Could you check a few things on this model? Use its own coordinates, in mm. A direction names the side the tool comes from. Round coordinates to 2 decimals unless told otherwise and drop trailing zeros. Write each loop counter-clockwise with the first axis right and the second up, starting at its lowest first coordinate (ties: lowest second). Pieces come first, ordered by that corner, then holes. Notation, with made-up numbers: (-15, 49.5) -> (0, 49.5) arc R5 ccw to (0, 56.5) -> close; hole circle Ø4 at (54, 45.25). An arc over 180 degrees is marked (long way). Answer as CSV lines item,"result". Start each with the question number.
Q1. Imagine slicing it at A-A on x = -23.25. Please give me the cut outline in (y, z).
Q2. For faces 1 (the cylindrical face through (39.43, 24.82, 20.07)), 2 (the cylindrical face through (-28.319, -28.778, 29.944)), 3 (the flat face through (-68.2, 0, -46)), which set-ups out of +Z, -Z, +X, -X, +Y, -Y let a thin tool reach every point of the face, with its end or its side?
Q3. Will these pins go through, and if not, where does the flat tip stop? pin 1 Ø19.5 at (x, y) = (23.25, 23.25) entering from -Z; pin 2 Ø9 at (x, z) = (42.5, -4.2) entering from +Y; pin 3 Ø7 at (x, y) = (-23.25, -23.25) entering from +Z; pin 4 Ø7.5 at (y, z) = (23.25, -63) entering from -X.
Q4. If we mould it in two halves opening along Y, with no side actions, what happens to faces 4 (the cylindrical face through (59.243, 22.53, -24.456)), 5 (the flat face through (68.2, 0, 51)), 6 (the cylindrical face through (-59, 26.32, 20.07)), 7 (the conical face through (-42.183, 13.562, -4.698))? For each: pulls with the +Y half, pulls with the -Y half, needs draft (parallel to the pull), parting line crosses it, or undercut.
Q5. Imagine slicing it at B-B on x = -57. Give the number of separate pieces and of enclosed holes in the cut face, and give its area (3 significant figures).
Q6. If I drill on line 1 (Y direction, x = 23.25, z = 19); line 2 (Z direction, x = 58, y = -23.25); line 3 (Z direction, x = -42, y = 20), over which ranges is the centre line in solid material (lowest first)? Write a range as [from, to].
Q7. Imagine slicing it at C-C on x = -7.5. Please give me the cut outline in (y, z).
from build123d import *

# Parameters (mm, degrees)
BOSS_EXTRUDE1_DEPTH      = 35
BOSS_EXTRUDE1_DEPTH_BACK = 35
SKETCH2_W                = 36
SKETCH2_H                = 20
HOLE1_D                  = 6.647
HOLE1_DEPTH              = 19.414509714
HOLE1_CSINK_D            = 8
HOLE1_CSINK_ANGLE        = 90
HOLE1_TIP                = 1.91882362
HOLE2_D                  = 6.647
HOLE2_DEPTH              = 19.414509714
HOLE2_CSINK_D            = 8
HOLE2_CSINK_ANGLE        = 90
HOLE2_TIP                = 1.91882362
HOLE3_D                  = 6.647
HOLE3_DEPTH              = 19.414509714
HOLE3_CSINK_D            = 8
HOLE3_CSINK_ANGLE        = 90
HOLE3_TIP                = 1.91882362
SKETCH26_R               = 10
CUT_EXTRUDE1_DEPTH       = 150
SKETCH27_R               = 10
CUT_EXTRUDE2_DEPTH       = 150
SKETCH28_W               = 177
SKETCH28_H               = 190
CUT_EXTRUDE3_DEPTH       = 70
CUT_EXTRUDE3_DEPTH_BACK  = 70
SKETCH29_R               = 4
CUT_EXTRUDE4_DEPTH       = 17.5
M8_TAPPED_HOLE1_D        = 6.8
M8_TAPPED_HOLE1_DEPTH    = 19.75
M8_TAPPED_HOLE1_TIP      = 2.042926105


with BuildPart() as part:
    # Sketch1 → Boss-Extrude1 (new body, two sides)
    with BuildSketch(Plane(origin=(0, 0, 0), x_dir=(1, 0, 0), z_dir=(0, 1, 0))) as boss_extrude1_sk:
        with BuildLine():
            Line((-68.5, -71), (-35.25, -71))
            Line((-35.25, -71), (-35.25, -34))
            Line((-35.25, -34), (35.25, -34))
            Line((35.25, -34), (35.25, -71))
            Line((35.25, -71), (68.5, -71))
            Line((68.5, -71), (68.5, 79))
            Line((68.5, 79), (35.25, 79))
            Line((35.25, 79), (35.25, 0))
            ThreePointArc((35.25, 0), (34, -1.25), (32.75, 0))
            Line((32.75, 0), (-32.75, 0))
            ThreePointArc((-32.75, 0), (-34, -1.25), (-35.25, 0))
            Line((-35.25, 0), (-35.25, 79))
            Line((-35.25, 79), (-68.5, 79))
            Line((-68.5, 79), (-68.5, -71))
        make_face()
    extrude(amount=BOSS_EXTRUDE1_DEPTH)
    extrude(boss_extrude1_sk.sketch, amount=-BOSS_EXTRUDE1_DEPTH_BACK)

    # Sketch2 → Cut-Revolve1 (revolve, cut)
    with BuildSketch(Plane(origin=(0, 0, 0), x_dir=(0, 0, -1), z_dir=(1, 0, 0))):
        with Locations((-17, 10)):
            Rectangle(SKETCH2_W, SKETCH2_H)
    revolve(axis=Axis((0, 0, -1), (0, 0, 1)), mode=Mode.SUBTRACT)

    # Sketch3 → Cut-Revolve2 (revolve, cut)
    with BuildSketch(Plane(origin=(-23.25, 0, 0), x_dir=(0, 0, -1), z_dir=(1, 0, 0))):
        Polygon((-34, 23.25), (-34, 30.75), (-26, 30.75), (-26, 27.75), (0, 27.75), (0, 23.25), align=None)
    revolve(axis=Axis((-23.25, 23.25, 0), (0, 0, 1)), mode=Mode.SUBTRACT)

    # Sketch4 → Cut-Revolve3 (revolve, cut)
    with BuildSketch(Plane(origin=(-23.25, 0, 0), x_dir=(0, 0, -1), z_dir=(1, 0, 0))):
        Polygon((-34, -23.25), (-34, -15.75), (-26, -15.75), (-26, -18.75), (0, -18.75), (0, -23.25), align=None)
    revolve(axis=Axis((-23.25, -23.25, 0), (0, 0, 1)), mode=Mode.SUBTRACT)

    # Sketch5 → Cut-Revolve4 (revolve, cut)
    with BuildSketch(Plane(origin=(23.25, 0, 0), x_dir=(0, 0, -1), z_dir=(1, 0, 0))):
        Polygon((-34, 23.25), (-34, 30.75), (-26, 30.75), (-26, 27.75), (0, 27.75), (0, 23.25), align=None)
    revolve(axis=Axis((23.25, 23.25, 0), (0, 0, 1)), mode=Mode.SUBTRACT)

    # Sketch6 → Cut-Revolve5 (revolve, cut)
    with BuildSketch(Plane(origin=(23.25, 0, 0), x_dir=(0, 0, -1), z_dir=(1, 0, 0))):
        Polygon((-34, -23.25), (-34, -15.75), (-26, -15.75), (-26, -18.75), (0, -18.75), (0, -23.25), align=None)
    revolve(axis=Axis((23.25, -23.25, 0), (0, 0, 1)), mode=Mode.SUBTRACT)

    # Hole1
    with Locations(Plane(origin=(0, 35, 0), x_dir=(1, 0, 0), z_dir=(0, 1, 0))):
        with Locations((42.5, -18.8)):
            CounterSinkHole(HOLE1_D / 2, HOLE1_CSINK_D / 2, depth=HOLE1_DEPTH, counter_sink_angle=HOLE1_CSINK_ANGLE)
            with Locations((0, 0, -(HOLE1_DEPTH + HOLE1_TIP / 2))):  # 120° drill point
                Cone(0, HOLE1_D / 2, HOLE1_TIP, mode=Mode.SUBTRACT)

    # Hole2
    with Locations(Plane(origin=(0, 35, 0), x_dir=(1, 0, 0), z_dir=(0, 1, 0))):
        with Locations((-42.5, -18.8)):
            CounterSinkHole(HOLE2_D / 2, HOLE2_CSINK_D / 2, depth=HOLE2_DEPTH, counter_sink_angle=HOLE2_CSINK_ANGLE)
            with Locations((0, 0, -(HOLE2_DEPTH + HOLE2_TIP / 2))):  # 120° drill point
                Cone(0, HOLE2_D / 2, HOLE2_TIP, mode=Mode.SUBTRACT)

    # Sketch11 → Cut-Revolve6 (revolve, cut)
    with BuildSketch(Plane.XY.offset(18.8)):
        Polygon((48.5, 23.25), (50.41882362, 26.5735), (67.8235, 26.5735), (68.5, 27.25), (68.5, 23.25), align=None)
    revolve(axis=Axis((68.5, 23.25, 18.8), (-1, 0, 0)), mode=Mode.SUBTRACT)

    # Sketch12 → Cut-Revolve7 (revolve, cut)
    with BuildSketch(Plane.XY.offset(18.8)):
        Polygon((48.5, -23.25), (50.41882362, -19.9265), (67.8235, -19.9265), (68.5, -19.25), (68.5, -23.25), align=None)
    revolve(axis=Axis((68.5, -23.25, 18.8), (-1, 0, 0)), mode=Mode.SUBTRACT)

    # Sketch13 → Cut-Revolve8 (revolve, cut)
    with BuildSketch(Plane.XY.offset(18.8)):
        Polygon((-68.5, 23.25), (-68.5, 27.25), (-67.8235, 26.5735), (-50.41882362, 26.5735), (-48.5, 23.25), align=None)
    revolve(axis=Axis((-48.5, 23.25, 18.8), (-1, 0, 0)), mode=Mode.SUBTRACT)

    # Sketch14 → Cut-Revolve9 (revolve, cut)
    with BuildSketch(Plane.XY.offset(18.8)):
        Polygon((-68.5, -23.25), (-68.5, -19.25), (-67.8235, -19.9265), (-50.41882362, -19.9265), (-48.5, -23.25), align=None)
    revolve(axis=Axis((-48.5, -23.25, 18.8), (-1, 0, 0)), mode=Mode.SUBTRACT)

    # Hole3
    with Locations(Plane(origin=(0, 35, 0), x_dir=(1, 0, 0), z_dir=(0, 1, 0))):
        with Locations((42.5, 27.7)):
            CounterSinkHole(HOLE3_D / 2, HOLE3_CSINK_D / 2, depth=HOLE3_DEPTH, counter_sink_angle=HOLE3_CSINK_ANGLE)
            with Locations((0, 0, -(HOLE3_DEPTH + HOLE3_TIP / 2))):  # 120° drill point
                Cone(0, HOLE3_D / 2, HOLE3_TIP, mode=Mode.SUBTRACT)

    # Sketch17 → Cut-Revolve10 (revolve, cut)
    with BuildSketch(Plane.XY.offset(-27.7)):
        Polygon((-42.5, 35), (-38.5, 35), (-39.1765, 34.3235), (-39.1765, 15.585490286), (-42.5, 13.666666667), align=None)
    revolve(axis=Axis((-42.5, 13.666666667, -27.7), (0, 1, 0)), mode=Mode.SUBTRACT)

    # Sketch18 → Cut-Revolve11 (revolve, cut)
    with BuildSketch(Plane.XY.offset(-27.7)):
        Polygon((48.5, 23.25), (50.41882362, 26.5735), (67.8235, 26.5735), (68.5, 27.25), (68.5, 23.25), align=None)
    revolve(axis=Axis((68.5, 23.25, -27.7), (-1, 0, 0)), mode=Mode.SUBTRACT)

    # Sketch19 → Cut-Revolve12 (revolve, cut)
    with BuildSketch(Plane.XY.offset(-27.7)):
        Polygon((48.5, -23.25), (50.41882362, -19.9265), (67.8235, -19.9265), (68.5, -19.25), (68.5, -23.25), align=None)
    revolve(axis=Axis((68.5, -23.25, -27.7), (-1, 0, 0)), mode=Mode.SUBTRACT)

    # Sketch20 → Cut-Revolve13 (revolve, cut)
    with BuildSketch(Plane.XY.offset(-27.7)):
        Polygon((-68.5, 23.25), (-68.5, 27.25), (-67.8235, 26.5735), (-50.41882362, 26.5735), (-48.5, 23.25), align=None)
    revolve(axis=Axis((-48.5, 23.25, -27.7), (-1, 0, 0)), mode=Mode.SUBTRACT)

    # Sketch21 → Cut-Revolve14 (revolve, cut)
    with BuildSketch(Plane.XY.offset(-27.7)):
        Polygon((-68.5, -23.25), (-68.5, -19.25), (-67.8235, -19.9265), (-50.41882362, -19.9265), (-48.5, -23.25), align=None)
    revolve(axis=Axis((-48.5, -23.25, -27.7), (-1, 0, 0)), mode=Mode.SUBTRACT)

    # Sketch22 → Cut-Revolve15 (revolve, cut)
    with BuildSketch(Plane.XY.offset(-63)):
        Polygon((-68.5, 23.25), (-68.5, 27.25), (-67.8235, 26.5735), (-50.41882362, 26.5735), (-48.5, 23.25), align=None)
    revolve(axis=Axis((-48.5, 23.25, -63), (-1, 0, 0)), mode=Mode.SUBTRACT)

    # Sketch23 → Cut-Revolve16 (revolve, cut)
    with BuildSketch(Plane.XY.offset(-63)):
        Polygon((-68.5, -23.25), (-68.5, -19.25), (-67.8235, -19.9265), (-50.41882362, -19.9265), (-48.5, -23.25), align=None)
    revolve(axis=Axis((-48.5, -23.25, -63), (-1, 0, 0)), mode=Mode.SUBTRACT)

    # Sketch24 → Cut-Revolve17 (revolve, cut)
    with BuildSketch(Plane.XY.offset(37)):
        Polygon((-68.5, 23.25), (-68.5, 27.25), (-67.8235, 26.5735), (-50.41882362, 26.5735), (-48.5, 23.25), align=None)
    revolve(axis=Axis((-48.5, 23.25, 37), (-1, 0, 0)), mode=Mode.SUBTRACT)

    # Sketch25 → Cut-Revolve18 (revolve, cut)
    with BuildSketch(Plane.XY.offset(37)):
        Polygon((-68.5, -23.25), (-68.5, -19.25), (-67.8235, -19.9265), (-50.41882362, -19.9265), (-48.5, -23.25), align=None)
    revolve(axis=Axis((-48.5, -23.25, 37), (-1, 0, 0)), mode=Mode.SUBTRACT)

    # Sketch26 → Cut-Extrude1 (cut)
    with BuildSketch(Plane.XY.offset(-79)):
        with Locations((52, 0)):
            Circle(SKETCH26_R)
    extrude(amount=CUT_EXTRUDE1_DEPTH, mode=Mode.SUBTRACT)

    # Sketch27 → Cut-Extrude2 (cut)
    with BuildSketch(Plane.XY.offset(-79)):
        with Locations((-52, 0)):
            Circle(SKETCH27_R)
    extrude(amount=CUT_EXTRUDE2_DEPTH, mode=Mode.SUBTRACT)

    # Sketch28 → Cut-Extrude3 (cut, two sides)
    with BuildSketch(Plane(origin=(0, 0, 0), x_dir=(1, 0, 0), z_dir=(0, 1, 0))) as cut_extrude3_sk:
        with Locations((0, 4)):
            Rectangle(SKETCH28_W, SKETCH28_H)
        Polygon((-68.5, 18), (-68.2, 18), (-68.2, -9), (-68.5, -9), (-68.5, -47), (-68.2, -47), (-68.2, -71), (68.2, -71), (68.2, -31), (68.5, -31), (68.5, -9), (68.2, -9), (68.2, 18), (68.5, 18), (68.5, 40), (68.2, 40), (68.2, 79), (-68.5, 79), (-68.5, 52), (-68.2, 52), (-68.2, 40), (-68.5, 40), align=None, mode=Mode.SUBTRACT)
    extrude(amount=CUT_EXTRUDE3_DEPTH, mode=Mode.SUBTRACT)
    extrude(cut_extrude3_sk.sketch, amount=-CUT_EXTRUDE3_DEPTH_BACK, mode=Mode.SUBTRACT)

    # Sketch29 → Cut-Extrude4 (cut)
    with BuildSketch(Plane(origin=(0, 35, 0), x_dir=(1, 0, 0), z_dir=(0, 1, 0))):
        with Locations((-42.5, 42.7)):
            Circle(SKETCH29_R)
        with Locations((42.5, -33.8)):
            Circle(SKETCH29_R)
    extrude(amount=-CUT_EXTRUDE4_DEPTH, mode=Mode.SUBTRACT)

    # M8 Tapped Hole1
    with Locations(Plane(origin=(0, 35, 0), x_dir=(1, 0, 0), z_dir=(0, 1, 0))):
        with Locations((-42.5, 4.2), (42.5, 4.2)):
            Hole(M8_TAPPED_HOLE1_D / 2, depth=M8_TAPPED_HOLE1_DEPTH)
            with Locations((0, 0, -(M8_TAPPED_HOLE1_DEPTH + M8_TAPPED_HOLE1_TIP / 2))):  # 118° drill point
                Cone(0, M8_TAPPED_HOLE1_D / 2, M8_TAPPED_HOLE1_TIP, mode=Mode.SUBTRACT)


solid = part.part
Checks:
1,outline,"(-35, 0) -> (-27.75, 0) -> (-27.75, 26) -> (-30.75, 26) -> (-30.75, 34) -> (-35, 34) -> close; (-18.75, 0) -> (18.75, 0) -> (18.75, 26) -> (15.75, 26) -> (15.75, 34) -> (-15.75, 34) -> (-15.75, 26) -> (-18.75, 26) -> close; (27.75, 0) -> (35, 0) -> (35, 34) -> (30.75, 34) -> (30.75, 26) -> (27.75, 26) -> close"
2,face 1,"+Y"
2,face 2,"+Z"
2,face 3,"-X, +Y, -Y"
3,pin 1,"z = 0"
3,pin 2,"y = 35"
3,pin 3,"through"
3,pin 4,"x = -68.25"
4,face 4,"undercut"
4,face 5,"needs draft"
4,face 6,"undercut"
4,face 7,"pulls with the +Y half"
5,separate pieces,"2"
5,enclosed holes,"8"
5,area,"7,620 mm^2"
6,line 1,"[-35, -27.75], [-18.75, 18.75], [27.75, 35]"
6,line 2,"[-79, -31.02], [-24.38, 15.48], [22.12, 71]"
6,line 3,"[-79, -46.67], [-38.73, -30.99], [-24.41, -7.56], [-0.84, 15.51], [22.09, 71]"
7,outline,"(-35, 0) -> (-18.54, 0) -> (-18.54, 34) -> (-35, 34) -> close; (18.54, 0) -> (35, 0) -> (35, 34) -> (18.54, 34) -> close"
